The listing builds one solid part. Answer for the finished solid, in the listing's coordinates (mm). Give positions to 0.01 mm unless a question says otherwise; leave off trailing zeros. Write each loop counter-clockwise with the first axis right and the second up, starting at its lowest first coordinate (ties: lowest second). Pieces come first, ordered by that corner, then holes. Notation, with made-up numbers: (-20, 15.25) - (15, 15.25) arc R16 cw to (15, 23.25) - close; hole circle Ø7 at (39.25, -13). An arc over 180 degrees is marked (long way). Answer in a Markdown table with one row per item. Add a question column.
from build123d import *

# Parameters (mm, degrees)
BASE_DEPTH         = 5
CUT_EXTRUDE1_DEPTH = 260.326049598


with BuildPart() as part:
    # Sketch1 → base (new body)
    with BuildSketch(Plane.XY):
        with BuildLine():
            Line((-45, 120), (-45, 70))
            Line((-45, 70), (-20, 70))
            ThreePointArc((-20, 70), (-5.857864376, 64.142135624), (0, 50))
            Line((0, 50), (0, 20))
            ThreePointArc((0, 20), (5.857864376, 5.857864376), (20, 0))
            Line((20, 0), (123.724055084, 0))
            ThreePointArc((123.724055084, 0), (133.546443389, 2.578154863), (140.836467877, 9.647931201))
            Line((140.836467877, 9.647931201), (193.502928783, 96.707845203))
            ThreePointArc((193.502928783, 96.707845203), (173.694009897, 160.933287114), (112.183133888, 133.846153846))
            ThreePointArc((112.183133888, 133.846153846), (104.920383724, 123.827849199), (93.153415616, 120))
            Line((93.153415616, 120), (-45, 120))
        make_face()
    extrude(amount=BASE_DEPTH)

    # Sketch2 → Cut-Extrude1 (cut, through all)
    with BuildSketch(Plane.XY.offset(5)):
        with BuildLine():
            Line((93.153415616, 105), (-30, 105))
            Line((-30, 105), (-30, 85))
            Line((-30, 85), (-20, 85))
            ThreePointArc((-20, 85), (4.748737342, 74.748737342), (15, 50))
            Line((15, 50), (15, 20))
            ThreePointArc((15, 20), (16.464466094, 16.464466094), (20, 15))
            Line((20, 15), (123.724055084, 15))
            ThreePointArc((123.724055084, 15), (126.179652161, 15.644538716), (128.002158282, 17.4119828))
            Line((128.002158282, 17.4119828), (180.668619189, 104.471896802))
            ThreePointArc((180.668619189, 104.471896802), (167.462673265, 147.288858076), (126.455422592, 129.230769231))
            ThreePointArc((126.455422592, 129.230769231), (113.745609805, 111.698736098), (93.153415616, 105))
        make_face()
    extrude(amount=-CUT_EXTRUDE1_DEPTH, mode=Mode.SUBTRACT)


solid = part.part
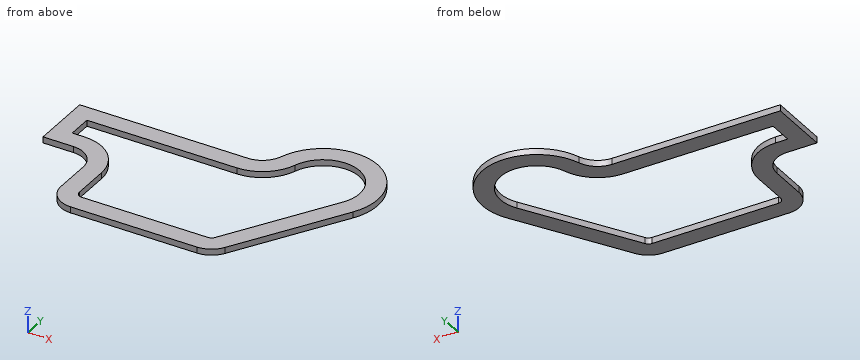
1. Straight lines are drawn through the part: L1, parallel to Y at x = 52.5, z = 1.1; L2, parallel to Y at x = 15.5, z = 2.45; L3, parallel to X at y = 110, z = 3.25. For each, find the intervals that lie inside material, in ascending order. Write a range as [from, to].
2. Section C-C (z = 1.2) is taken. Give the vertices of the cut face in (x, y).
3. Section A-A (x = 50.5) is taken. Give the vertices of the cut face in (y, z), and give its area (3 significant figures).
4. Section B-B (y = 138) is taken. Give the vertices of the cut face in (x, z), and give its area (3 significant figures).
5. Given pin 1 Ø3 at (y, z) = (132, 1) entering from -X; pin 2 Ø1.5 at (x, z) = (-24.5, 2) entering from +Y; pin 3 Ø2.5 at (y, z) = (33.5, 3) entering from +X, each flat-ended and moving along its own axis, determine where each tip first touches the part or whether it passes through.
Geometry check:
| question | item | result |
|---|---|---|
| 1 | L1 | [0, 15], [105, 120] |
| 1 | L2 | [0.51, 17.82], [105, 120] |
| 1 | L3 | [-45, 111.18], [183.28, 198.87] |
| 2 | outline | (-45, 70) - (-20, 70) arc R20 cw to (0, 50) - (0, 20) arc R20 ccw to (20, 0) - (123.72, 0) arc R20 ccw to (140.84, 9.65) - (193.5, 96.71) arc R45 ccw (long way) to (112.18, 133.85) arc R20 cw to (93.15, 120) - (-45, 120) - close; hole (-30, 85) - (-20, 85) arc R35 cw to (15, 50) - (15, 20) arc R5 ccw to (20, 15) - (123.72, 15) arc R5 ccw to (128, 17.41) - (180.67, 104.47) arc R30 ccw (long way) to (126.46, 129.23) arc R35 cw to (93.15, 105) - (-30, 105) - close |
| 3 | outline | (0, 0) - (15, 0) - (15, 5) - (0, 5) - close; (105, 0) - (120, 0) - (120, 5) - (105, 5) - close |
| 3 | area | 150 mm² |
| 4 | outline | (113.76, 0) - (131, 0) - (131, 5) - (113.76, 5) - close; (179, 0) - (196.24, 0) - (196.24, 5) - (179, 5) - close |
| 4 | area | 172 mm² |
| 5 | pin 1 | x = 110.75 |
| 5 | pin 2 | y = 120 |
| 5 | pin 3 | x = 156.02 |
